```python
from build123d import *

# Parameters (mm, degrees)
SKETCH1_W           = 304.8
SKETCH1_H           = 304.8
BOSS_EXTRUDE1_DEPTH = 6.35
CUT_EXTRUDE2_DEPTH  = 6.35
SKETCH3_R           = 1.190625
SKETCH3_R_2         = 1.3890625
CUT_EXTRUDE3_DEPTH  = 335.039575687
FILLET2_R           = 2.54


with BuildPart() as part:
    # Sketch1 → Boss-Extrude1 (new body)
    with BuildSketch(Plane(origin=(0, 0, 0), x_dir=(1, 0, 0), z_dir=(0, 1, 0))):
        with Locations((152.4, 152.4)):
            Rectangle(SKETCH1_W, SKETCH1_H)
    extrude(amount=BOSS_EXTRUDE1_DEPTH)

    # Sketch2 → Cut-Extrude2 (cut)
    with BuildSketch(Plane(origin=(0, 6.35, 0), x_dir=(1, 0, 0), z_dir=(0, 1, 0))):
        Polygon((136.525, 304.8), (136.525, 295.275), (0, 295.275), (0, 0), (304.8, 0), (304.8, 304.8), align=None)
    extrude(amount=-CUT_EXTRUDE2_DEPTH, mode=Mode.SUBTRACT)

    # Sketch3 → Cut-Extrude3 (cut, through all)
    with BuildSketch(Plane(origin=(0, 6.35, 0), x_dir=(1, 0, 0), z_dir=(0, 1, 0))):
        with Locations(Location((6.35, 299.92676377, 0), (0, 0, 270))):
            Circle(SKETCH3_R)
        with Locations(Location((25.4, 299.92676377, 0), (0, 0, 270))):
            Circle(SKETCH3_R)
        with Locations(Location((114.3, 299.92676377, 0), (0, 0, 270))):
            Circle(SKETCH3_R_2)
        with Locations(Location((127, 299.92676377, 0), (0, 0, 270))):
            Circle(SKETCH3_R_2)
    extrude(amount=-CUT_EXTRUDE3_DEPTH, mode=Mode.SUBTRACT)

    # Fillet2
    fillet2_edges = [part.edges().sort_by_distance(p)[0] for p in [
        (136.525, 3.175, -304.8),
    ]]
    fillet(fillet2_edges, radius=FILLET2_R)


solid = part.part
```
Check sheet for the modelled part. Datum: model origin and axes. Units: mm. Round coordinates to 2 decimals unless told otherwise and drop trailing zeros. Order: outer loops, then holes, each group sorted by start corner. A loop starts at its lowest first (then second) coordinate and runs counter-clockwise, first axis right, second up. Notation, with made-up numbers: (14.25, -31.5) - (42.25, -31.5) arc R35 ccw to (42.25, 4.5) - close; hole circle Ø4 at (63.25, 55.25). An arc over 180 degrees is marked (long way). Answer as CSV lines item,"result". Start each with the question number.
1) Section check B-B (z = -300). Record the cut outline in (x, y) (3 decimals), then the cut area to 3 significant figures.
2) Scan lines: probe 1 along X at (y, z) = (4, -300) (3 decimals); probe 2 along Z at (x, y) = (128, 2) (3 decimals); probe 3 along X at (y, z) = (3.5, -303.5). Record each from-to range of solid material in increasing order.
3) Draft check along X on faces 1 (the face through (114.717, 3.219, -298.602)), 2 (the face through (136.525, 3, -299)), 3 (the face through (0, 3, -300)), 4 (the face through (67, 6.35, -300)). Enter one of: +X half, -X half, draft (parallel to the pull), parting line (faces both ways), or undercut.
4) Section check D-D (x = 6.35). Record the cut outline in (y, z) (3 decimals), then the cut area to 3 significant figures.
5) Section check A-A (x = 114.3). Record the cut outline in (y, z) (3 decimals), then the cut area to 3 significant figures.
6) Section check C-C (y = 5). Record the cut outline in (x, z) (3 decimals).
Determined:
1,outline,"(0, 0) - (5.162, 0) - (5.162, 6.35) - (0, 6.35) - close; (7.538, 0) - (24.212, 0) - (24.212, 6.35) - (7.538, 6.35) - close; (26.588, 0) - (112.913, 0) - (112.913, 6.35) - (26.588, 6.35) - close; (115.687, 0) - (125.613, 0) - (125.613, 6.35) - (115.687, 6.35) - close; (128.387, 0) - (136.525, 0) - (136.525, 6.35) - (128.387, 6.35) - close"
1,area,"802 mm^2"
2,probe 1,"0 to 5.162, 7.538 to 24.212, 26.588 to 112.913, 115.687 to 125.613, 128.387 to 136.525"
2,probe 2,"-304.8 to -300.891, -298.963 to -295.275"
2,probe 3,"0 to 136.2"
3,face 1,"undercut"
3,face 2,"+X half"
3,face 3,"-X half"
3,face 4,"draft"
4,outline,"(0, -304.8) - (6.35, -304.8) - (6.35, -301.117) - (0, -301.117) - close; (0, -298.736) - (6.35, -298.736) - (6.35, -295.275) - (0, -295.275) - close"
4,area,"45.4 mm^2"
5,outline,"(0, -304.8) - (6.35, -304.8) - (6.35, -301.316) - (0, -301.316) - close; (0, -298.538) - (6.35, -298.538) - (6.35, -295.275) - (0, -295.275) - close"
5,area,"42.8 mm^2"
6,outline,"(0, -304.8) - (133.985, -304.8) arc R2.54 ccw to (136.525, -302.26) - (136.525, -295.275) - (0, -295.275) - close; hole circle Ø2.381 at (6.35, -299.927); hole circle Ø2.381 at (25.4, -299.927); hole circle Ø2.778 at (114.3, -299.927); hole circle Ø2.778 at (127, -299.927)"
